from build123d import *

# Parameters (mm, degrees)
F0_R     = 11
F1_DEPTH = 100
F2_T     = -2
F3_R     = 3
F4_R     = 1


with BuildPart() as f1:
    # F0 (on Top) → F1 (new body)
    with BuildSketch(Plane.XY):
        Circle(F0_R)
    extrude(amount=F1_DEPTH)

    # F2
    f2_openings = [f1.faces().sort_by_distance(p)[0] for p in [
        (0, 0, 100),
    ]]
    offset(amount=F2_T, openings=f2_openings)

    # F3
    f3_edges = [f1.edges().sort_by_distance(p)[0] for p in [
        (-11, 0, 0),
    ]]
    fillet(f3_edges, radius=F3_R)

    # F4
    f4_edges = [f1.edges().sort_by_distance(p)[0] for p in [
        (-11, 0, 100),
    ]]
    fillet(f4_edges, radius=F4_R)


solid = f1.part
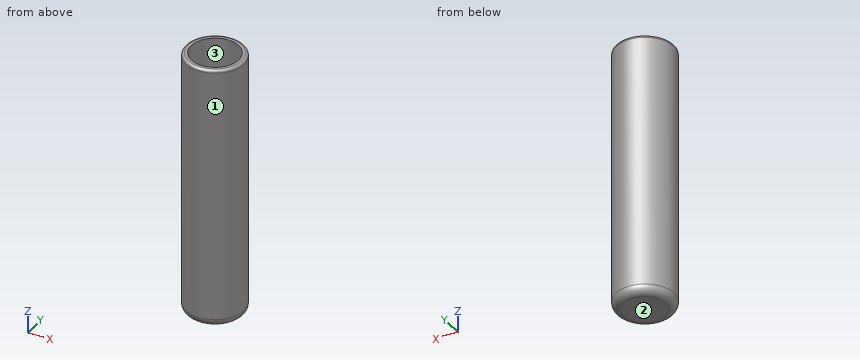
Can you work these out from the model? Positions are in its coordinate system, mm. Face numbers are marked on the shaded views. Round coordinates to 2 decimals unless told otherwise and drop trailing zeros. Loops run counter-clockwise (first coordinate to the right, second up) from the corner with the lowest first, then second, coordinate; pieces in that order, holes last. Notation, with made-up numbers: (34, 59.25) - (48, 59.25) arc R37 cw to (48, 96.25) - close; hole circle Ø3 at (9.25, 41.25). An arc over 180 degrees is marked (long way). Answer in a Markdown table with one row per item. Add a question column.
Q1. I want a section at A-A on x = 0. List the corners of the cut face in (y, z) for me.
Q2. I want a section at C-C on z = 62. List the corners of the cut face in (x, y) for me.
Q3. We'd pull the mould along Y, two halves only. Please class the marked faces 1, 2 and 3: pulls with the +Y half, pulls with the -Y half, needs draft (parallel to the pull), parting line crosses it, or undercut.
Q4. For pin 1 Ø2 at (x, y) = (4, -3.5) entering from +Z; pin 2 Ø1 at (x, y) = (5, 7.5) entering from -Z; pin 3 Ø6 at (x, z) = (-8.5, 68.5) entering from -Y, each with a flat end and sliding along its axis, tell me the tip position at first contact or that it passes through.
Q5. I need wall thicknesses on L1, parallel to X at y = -0.25, z = 66; L2, parallel to Y at x = 0.5, z = 65; L3, parallel to Z at x = -4.5, y = 4.25. Which ranges of each line are inside material? Lowest first, please.
A:
| question | item | result |
|---|---|---|
| 1 | outline | (-11, 3) arc R3 ccw to (-8, 0) - (8, 0) arc R3 ccw to (11, 3) - (11, 99) arc R1 ccw to (10, 100) - (9, 100) - (9, 2) - (-9, 2) - (-9, 100) - (-10, 100) arc R1 ccw to (-11, 99) - close |
| 2 | outline | circle Ø22 at (0, 0); hole circle Ø18 at (0, 0) |
| 3 | face 1 | parting line crosses it |
| 3 | face 2 | needs draft |
| 3 | face 3 | undercut |
| 4 | pin 1 | z = 2 |
| 4 | pin 2 | z = 0.04 |
| 4 | pin 3 | y = -9.53 |
| 5 | L1 | -11 to -9, 9 to 11 |
| 5 | L2 | -10.99 to -8.99, 8.99 to 10.99 |
| 5 | L3 | 0 to 2 |
